The listing builds one solid part. Answer for the finished solid, in the listing's coordinates (mm). A direction names the side the tool comes from. Coordinates: 2 decimals unless noted, no trailing zeros. Loops run counter-clockwise (first coordinate to the right, second up) from the corner with the lowest first, then second, coordinate; pieces in that order, holes last. Notation, with made-up numbers: (58.5, 70.25) - (64.5, 70.25) arc R22 ccw to (64.5, 104.25) - close; hole circle Ø5 at (0, -39.5). An arc over 180 degrees is marked (long way). Return JSON: item names as keys, results as strings. Group by question number.
1. Section C-C (y = 3.5) is taken. Write down the section's boundary in (x, z), and give its area (3 significant figures).
2. Which of the six approach directions +Z, -Z, +X, -X, +Y, -Y give full straight-line access (tool end or side, diameter ignored) to faces 4 (the face through (-1.66, 2.46, -0.37)), 5 (the face through (0, 6, 0))?
3. The mould has two halves that part along Z. Classify faces 1 (the face through (0.931, 2.761, 2.957)), 2 (the face through (0, 5, 0)), 3 (the face through (-1.33, 0, 1.33)): pulls with the +Z half, pulls with the -Z half, needs draft (parallel to the pull), parting line crosses it, or undercut.
4. Section A-A (z = 0) is taken. Write down the section's boundary in (x, y), and give its area (3 significant figures).
5. Section B-B (x = 0) is taken. Write down the section's boundary in (y, z), and give its area (3 significant figures).
6. Find the intervals of material crossed by line 1 along X through (y, z) = (1.65, 0); line 2 along Y through (x, z) = (-0.25, 1.5); line 3 along X through (y, z) = (4.6, -0.75), in increasing order.
7. This flat-tipped pin is pushed along its axis until it touches: P1, Ø1.7, axis at x = 0.5, z = 0.5, coming from the -Y side. Where does it stop, or does it pass through?
```python
from build123d import *

# Parameters (mm, degrees)
SKETCH_1_R      = 3.1
SKETCH_1_R_2    = 1.7
EXTRUDE_1_DEPTH = 5
SKETCH_2_R      = 3.1
EXTRUDE_2_DEPTH = 1
FILLET_1_R      = 0.4


with BuildPart() as part:
    # 草图1 → 凸台-拉伸1 (new body)
    with BuildSketch(Plane(origin=(0, 0, 0), x_dir=(1, 0, 0), z_dir=(0, 1, 0))):
        with Locations(Location((0, 0, 0), (0, 0, 270))):
            Circle(SKETCH_1_R)
        with Locations(Location((0, 0, 0), (0, 0, 270))):
            Circle(SKETCH_1_R_2, mode=Mode.SUBTRACT)
    extrude(amount=EXTRUDE_1_DEPTH)

    # 草图2 → 凸台-拉伸2 (add)
    with BuildSketch(Plane(origin=(0, 5, 0), x_dir=(1, 0, 0), z_dir=(0, 1, 0))):
        with Locations(Location((0, 0, 0), (0, 0, 270))):
            Circle(SKETCH_2_R)
    extrude(amount=EXTRUDE_2_DEPTH)

    # 圆角1
    fillet_1_edges = [part.edges().sort_by_distance(p)[0] for p in [
        (0, 6, -3.1),
    ]]
    fillet(fillet_1_edges, radius=FILLET_1_R)


solid = part.part
```
The answers:
{
 "1": {"outline": "circle Ø6.2 at (0, 0); hole circle Ø3.4 at (0, 0)", "area": "21.1 mm2"},
 "2": {"face 4": "-Y", "face 5": "+Z, -Z, +X, -X, +Y"},
 "3": {"face 1": "parting line crosses it", "face 2": "undercut", "face 3": "needs draft"},
 "4": {"outline": "(-3.1, 0) - (-1.7, 0) - (-1.7, 5) - (1.7, 5) - (1.7, 0) - (3.1, 0) - (3.1, 5.6) arc R0.4 ccw to (2.7, 6) - (-2.7, 6) arc R0.4 ccw to (-3.1, 5.6) - close", "area": "20.1 mm2"},
 "5": {"outline": "(0, -3.1) - (5.6, -3.1) arc R0.4 ccw to (6, -2.7) - (6, 2.7) arc R0.4 ccw to (5.6, 3.1) - (0, 3.1) - (0, 1.7) - (5, 1.7) - (5, -1.7) - (0, -1.7) - close", "area": "20.1 mm2"},
 "6": {"line 1": "x = -3.1 to -1.7, 1.7 to 3.1", "line 2": "y = 5 to 6", "line 3": "x = -3.01 to -1.53, 1.53 to 3.01"},
 "7": {"P1": "stops at y = 5"}
}
